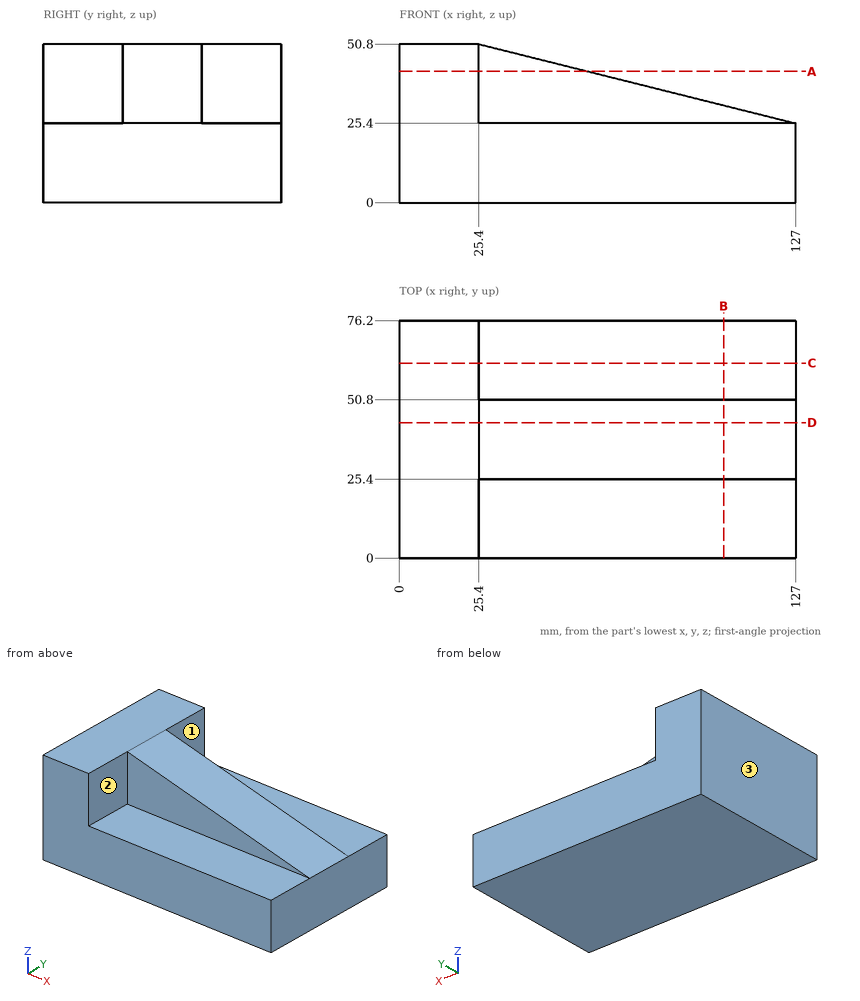
Geometry: see drawing. Coordinates: mm, zero at the bounding-box minimum. A direction names the side the tool comes from. Give positions to 0.01 mm unless a question says otherwise; leave off trailing zeros. Write each loop counter-clockwise with the first axis right and the second up, starting at its lowest first coordinate (ties: lowest second). Pieces come first, ordered by that corner, then holes. Notation, with made-up numbers: (-31, -30) -> (22, -30) arc R24 cw to (22, -9) -> close; hole circle Ø10 at (77, -29.75). An arc over 180 degrees is marked (long way). Use one line per item in the form item = value. Start each with the question number.
1) Set-up query: the marked faces 1, 2 and 3. Return all of +Z, -Z, +X, -X, +Y, -Y with unobstructed straight access to the full face (end or side cutting, diameter ignored); none if empty.
2) Pin query (flat end, axial travel): pin 1 (12.5 mm diameter, centred on y = 14.5, z = 33.5, fed in from +X); pin 2 (8 mm diameter, centred on x = 45, y = 38, fed in from +Z); pin 3 (12.5 mm diameter, centred on x = 92, z = 37, fed in from +Y); pin 4 (12.5 mm diameter, centred on x = 95, z = 42, fed in from -Y). Return the tip coordinate at first contact, or that it passes through.
3) Section query B-B on x = 104. Return the cut outline in (y, z), then the cut area to 3 significant figures.
4) Section query C-C on y = 62.5. Return the cut outline in (x, z).
5) Section query A-A on z = 42. Return the cut outline in (x, y), then the cut area to 3 significant figures.
6) Ray query, probe 1 along Z at (x, y) = (61, 19.5); probe 2 along Y at (x, z) = (51, 38). Return the intervals inside material, ascending. Write a range as from..to.
7) Section query D-D on y = 43.5. Return the cut outline in (x, z).
Outcome:
q1.face_1 = +Z, +X, +Y
q1.face_2 = +Z, +X, -Y
q1.face_3 = +Z, -Z, -X, +Y, -Y
q2.pin_1 = 25.4
q2.pin_2 = 46.9
q2.pin_3 = 50.8
q2.pin_4 = through
q3.outline = (0, 0) -> (76.2, 0) -> (76.2, 25.4) -> (50.8, 25.4) -> (50.8, 31.15) -> (25.4, 31.15) -> (25.4, 25.4) -> (0, 25.4) -> close
q3.area = 2,080 mm^2
q4.outline = (0, 0) -> (127, 0) -> (127, 25.4) -> (25.4, 25.4) -> (25.4, 50.8) -> (0, 50.8) -> close
q5.outline = (0, 0) -> (25.4, 0) -> (25.4, 25.4) -> (60.6, 25.4) -> (60.6, 50.8) -> (25.4, 50.8) -> (25.4, 76.2) -> (0, 76.2) -> close
q5.area = 2,830 mm^2
q6.probe_1 = 0..25.4
q6.probe_2 = 25.4..50.8
q7.outline = (0, 0) -> (127, 0) -> (127, 25.4) -> (25.4, 50.8) -> (0, 50.8) -> close
